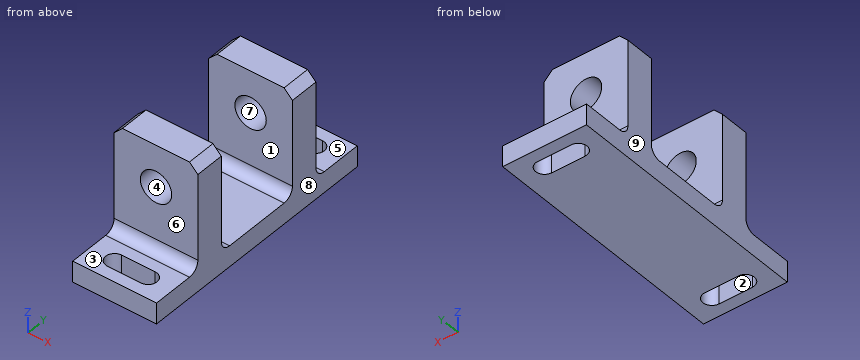
```python
from build123d import *

# Parameters (mm, degrees)
F1_DEPTH = 12.7
F2_R     = 4.7625
F3_DEPTH = 44.7675
F5_DEPTH = 6.35
F6_SIZE  = 2.54


with BuildPart() as f1:
    # F0 (on Right) → F1 (new body, symmetric)
    with BuildSketch(Plane.YZ):
        with BuildLine():
            Line((-38.1, 0), (0, 0))
            Line((0, 0), (38.1, 0))
            Line((38.1, 0), (38.1, 6.35))
            Line((38.1, 6.35), (25.55875, 6.35))
            ThreePointArc((25.55875, 6.35), (23.313686, 7.279936), (22.38375, 9.525))
            Line((22.38375, 9.525), (22.38375, 38.1))
            Line((22.38375, 38.1), (13.49375, 38.1))
            Line((13.49375, 38.1), (13.49375, 9.525))
            ThreePointArc((13.49375, 9.525), (12.563814, 7.279936), (10.31875, 6.35))
            Line((10.31875, 6.35), (0, 6.35))
            Line((0, 6.35), (-10.31875, 6.35))
            ThreePointArc((-10.31875, 6.35), (-12.563814, 7.279936), (-13.49375, 9.525))
            Line((-13.49375, 9.525), (-13.49375, 38.1))
            Line((-13.49375, 38.1), (-22.38375, 38.1))
            Line((-22.38375, 38.1), (-22.38375, 9.525))
            ThreePointArc((-22.38375, 9.525), (-23.313686, 7.279936), (-25.55875, 6.35))
            Line((-25.55875, 6.35), (-38.1, 6.35))
            Line((-38.1, 6.35), (-38.1, 0))
        make_face()
    extrude(amount=F1_DEPTH, both=True)

    # F2 (on face) → F3 (cut, through all)
    with BuildSketch(Plane.XZ.offset(22.38375)):
        with Locations((0, 25.4)):
            Circle(F2_R)
    extrude(amount=-F3_DEPTH, mode=Mode.SUBTRACT)

    # F4 (on face) → F5 (cut, through all)
    with BuildSketch(Plane.XY.offset(6.35)):
        with BuildLine():
            ThreePointArc((-5.08, 34.45), (-7.78, 31.75), (-5.08, 29.05))
            Line((-5.08, 29.05), (5.08, 29.05))
            ThreePointArc((5.08, 29.05), (7.78, 31.75), (5.08, 34.45))
            Line((5.08, 34.45), (-5.08, 34.45))
        make_face()
        with BuildLine():
            ThreePointArc((-5.08, -29.05), (-7.78, -31.75), (-5.08, -34.45))
            Line((-5.08, -34.45), (0, -34.45))
            Line((0, -34.45), (0, -29.05))
            Line((0, -29.05), (-5.08, -29.05))
        make_face()
        with BuildLine():
            Line((0, -29.05), (0, -34.45))
            Line((0, -34.45), (5.08, -34.45))
            ThreePointArc((5.08, -34.45), (7.78, -31.75), (5.08, -29.05))
            Line((5.08, -29.05), (0, -29.05))
        make_face()
    extrude(amount=-F5_DEPTH, mode=Mode.SUBTRACT)

    # F6
    f6_edges = [f1.edges().sort_by_distance(p)[0] for p in [
        (12.7, -17.93875, 38.1),
        (12.7, 17.93875, 38.1),
        (-12.7, -17.93875, 38.1),
        (-12.7, 17.93875, 38.1),
    ]]
    chamfer(f6_edges, length=F6_SIZE)


solid = f1.part
```
Input: part model. Units: mm. Frame: model coordinates. Face numbers are marked on the shaded views. A direction names the side the tool comes from. Give positions to 0.01 mm unless a question says otherwise; leave off trailing zeros. Order: outer loops, then holes, each group sorted by start corner. A loop starts at its lowest first (then second) coordinate and runs counter-clockwise, first axis right, second up. Notation, with made-up numbers: (-27, 47.5) - (3, 47.5) arc R10 cw to (3, 66.5) - close; hole circle Ø3 at (-37, 85). An arc over 180 degrees is marked (long way). Use a Markdown table: item, result.
(1) Line query: line 1 (Y direction, x = 0, z = 2.5); line 2 (Z direction, x = 0, y = 16.75); line 3 (Y direction, x = 7.25, z = 10). Output: solid intervals per line, ascending. Write a range as from..to.
Computed values:
| item | result |
|---|---|
| line 1 | y = -38.1..-34.45, -29.05..29.05, 34.45..38.1 |
| line 2 | z = 0..20.64, 30.16..38.1 |
| line 3 | y = -22.38..-13.49, 13.49..22.38 |
(2) Pin query (flat end, axial travel): pin 1 (1.5 mm diameter, centred on y = 11, z = 16.5, fed in from +X); pin 2 (7.5 mm diameter, centred on x = 2.5, z = 25, fed in from +Y); pin 3 (14 mm diameter, centred on x = 3.5, y = 34, fed in from +Z); pin 4 (1.5 mm diameter, centred on x = -8.5, z = 21, fed in from -Y). Return the tip coordinate at first contact, or that it passes through.
Computed values:
| item | result |
|---|---|
| pin 1 | passes through |
| pin 2 | stops at y = 22.38 |
| pin 3 | stops at z = 6.35 |
| pin 4 | stops at y = -22.38 |
(3) Section query A-A (z = 25.4). Output: boundary loops of the cut face in (x, y), then the cut area to 3 significant figures.
Computed values:
| item | result |
|---|---|
| outline | (-12.7, -22.38) - (-4.76, -22.38) - (-4.76, -13.49) - (-12.7, -13.49) - close; (-12.7, 13.49) - (-4.76, 13.49) - (-4.76, 22.38) - (-12.7, 22.38) - close; (4.76, -22.38) - (12.7, -22.38) - (12.7, -13.49) - (4.76, -13.49) - close; (4.76, 13.49) - (12.7, 13.49) - (12.7, 22.38) - (4.76, 22.38) - close |
| area | 282 mm2 |
(4) Access query for the marked faces 1, 2, 3, 4 and 5. Directions: +Z, -Z, +X, -X, +Y, -Y. A direction counts if a zero-diameter tool reaches every point of the face in a straight line with its end or side. Return the directions, or none.
Computed values:
| item | result |
|---|---|
| face 1 | +Z, +X, -X |
| face 2 | +Z, -Z |
| face 3 | +Z, +X, -X, -Y |
| face 4 | +Y, -Y |
| face 5 | +Z, +X, -X, +Y |
(5) Section query C-C (z = 17.5). Output: boundary loops of the cut face in (x, y), then the cut area to 3 significant figures.
Computed values:
| item | result |
|---|---|
| outline | (-12.7, -22.38) - (12.7, -22.38) - (12.7, -13.49) - (-12.7, -13.49) - close; (-12.7, 13.49) - (12.7, 13.49) - (12.7, 22.38) - (-12.7, 22.38) - close |
| area | 452 mm2 |
(6) Section query D-D (y = 31.75). Output: boundary loops of the cut face in (x, z), then the cut area to 3 significant figures.
Computed values:
| item | result |
|---|---|
| outline | (-12.7, 0) - (-7.78, 0) - (-7.78, 6.35) - (-12.7, 6.35) - close; (7.78, 0) - (12.7, 0) - (12.7, 6.35) - (7.78, 6.35) - close |
| area | 62.5 mm2 |
(7) Draft query along X for the marked faces 6, 7, 8 and 9. Return one class per face: released by +X, released by -X, zero draft, split by the parting line, or undercut.
Computed values:
| item | result |
|---|---|
| face 6 | zero draft |
| face 7 | undercut |
| face 8 | released by +X |
| face 9 | released by -X |
(8) Section query B-B (x = 0). State how many separate pieces and enclosed holes the cut face has, then the cut area to 3 significant figures.
Computed values:
| item | result |
|---|---|
| separate pieces | 5 |
| enclosed holes | 0 |
| area | 819 mm2 |
